Input: part model. Units: mm. Frame: model coordinates. A direction names the side the tool comes from. Coordinates: 2 decimals unless noted, no trailing zeros. Write each loop counter-clockwise with the first axis right and the second up, starting at its lowest first coordinate (ties: lowest second). Pieces come first, ordered by that corner, then holes. Notation, with made-up numbers: M -17.5,39 L 38.5,39 A10 ccw 38.5,56 Z; hole C -23.5,42 d7. An arc over 180 degrees is marked long. Use CSV: the item, a comma, the result in double quotes.
```python
from build123d import *

# Parameters (mm, degrees)
SKETCH_1_W                  = 40
SKETCH_1_H                  = 47.1
EXTRUDE_1_DEPTH             = 10
HOLE_WIZARD_M4_1_AT_2_COUNT = 2
HOLE_WIZARD_M4_1_AT_2_PITCH = 32
HOLE_WIZARD_M5_1_D          = 4.2
HOLE_WIZARD_M5_1_DEPTH      = 12.4
HOLE_WIZARD_M5_1_TIP        = 1.2618073
CUT_EXTRUDE_1_REACH         = 34.475
SKETCH_8_W                  = 24
SKETCH_8_H                  = 27.1
FILLET_1_R                  = 3


with BuildPart() as part:
    # 草图1 → 凸台-拉伸1 (new body)
    with BuildSketch(Plane.XY):
        Rectangle(SKETCH_1_W, SKETCH_1_H)
    extrude(amount=EXTRUDE_1_DEPTH)

    # 草图4 → M4 螺纹孔1 (revolve, cut)
    with BuildSketch(Plane(origin=(-16, 23.55, 5), x_dir=(0, 0, 1), z_dir=(1, 0, 0))):
        Polygon((0, 0), (0, 11.091420021), (1.65, 10.1), (1.65, 0), align=None)
    hole_wizard_m4_1 = revolve(axis=Axis((-16, 29.9, 5), (0, -1, 0)), mode=Mode.SUBTRACT)

    # M4 螺纹孔1 at 2: M4 螺纹孔1 ×2
    with Locations(*[(i * HOLE_WIZARD_M4_1_AT_2_PITCH, 0, 0) for i in range(1, HOLE_WIZARD_M4_1_AT_2_COUNT)]):
        add(hole_wizard_m4_1, mode=Mode.SUBTRACT)

    # 镜向1: M4 螺纹孔1 across plane
    add(hole_wizard_m4_1.mirror(Plane.ZX), mode=Mode.SUBTRACT)

    # 镜向1 copy 1 sketch → 镜向1 copy 1 (revolve, cut)
    with BuildSketch(Plane(origin=(16, -23.55, 5), x_dir=(0, 0, 1), z_dir=(1, 0, 0))):
        Polygon((0, 0), (0, -11.091420021), (1.65, -10.1), (1.65, 0), align=None)
    revolve(axis=Axis((16, -29.9, 5), (0, -1, 0)), mode=Mode.SUBTRACT)

    # M5 螺纹孔1
    with Locations(Plane.XY.offset(10)):
        with Locations((0, 0)):
            Hole(HOLE_WIZARD_M5_1_D / 2, depth=HOLE_WIZARD_M5_1_DEPTH)
            with Locations((0, 0, -(HOLE_WIZARD_M5_1_DEPTH + HOLE_WIZARD_M5_1_TIP / 2))):  # 118° drill point
                Cone(0, HOLE_WIZARD_M5_1_D / 2, HOLE_WIZARD_M5_1_TIP, mode=Mode.SUBTRACT)

    # 切除-拉伸1: up to this face of the body (flat: up to its plane)
    cut_extrude_1_end = Plane(part.part.faces().sort_by_distance((0, -22.932067156, 0))[0])
    # 草图8 → 切除-拉伸1 (cut, up to the picked face)
    with BuildSketch(Plane.XY.offset(10), mode=Mode.PRIVATE) as cut_extrude_1_sk1:
        with Locations((20, 0)):
            Rectangle(SKETCH_8_W, SKETCH_8_H)
    cut_extrude_1_tool1 = split(extrude(cut_extrude_1_sk1.sketch, amount=-CUT_EXTRUDE_1_REACH, mode=Mode.PRIVATE), bisect_by=cut_extrude_1_end, keep=Keep.BOTH, mode=Mode.PRIVATE)
    cut_extrude_1 = cut_extrude_1_tool1.solids().sort_by(Axis((20, 0, 10), (0, 0, -1)))[0]
    add(cut_extrude_1, mode=Mode.SUBTRACT)

    # 镜向2: 切除-拉伸1 across plane
    add(cut_extrude_1.mirror(Plane(origin=(0, 0, 0), x_dir=(0, 0, 1), z_dir=(1, 0, 0))), mode=Mode.SUBTRACT)

    # 圆角1
    fillet_1_edges = [part.edges().sort_by_distance(p)[0] for p in [
        (8, 13.55, 5),
        (8, -13.55, 5),
        (-8, -13.55, 5),
        (-8, 13.55, 5),
    ]]
    fillet(fillet_1_edges, radius=FILLET_1_R)


solid = part.part
```
1. Section C-C (z = 7.5). Return loops of the section in (x, y).
Resolved:
outline,"M -20,-23.55 L 20,-23.55 L 20,-13.55 L 11,-13.55 A3 cw 8,-10.55 L 8,10.55 A3 cw 11,13.55 L 20,13.55 L 20,23.55 L -20,23.55 L -20,13.55 L -11,13.55 A3 cw -8,10.55 L -8,-10.55 A3 cw -11,-13.55 L -20,-13.55 Z; hole C 0,0 d4.2"
2. Section A-A (x = 0). Return loops of the section in (y, z), then the cut area to 3 significant figures.
Resolved:
outline,"M -23.55,0 L -2.1,0 L -2.1,10 L -23.55,10 Z; M 2.1,0 L 23.55,0 L 23.55,10 L 2.1,10 Z"
area,"429 mm^2"
3. Section D-D (x = 16). Return loops of the section in (y, z), then the cut area to 3 significant figures.
Resolved:
outline,"M -23.55,0 L -13.55,0 L -13.55,3.35 L -23.55,3.35 Z; M -23.55,6.65 L -13.55,6.65 L -13.55,10 L -23.55,10 Z; M 13.55,0 L 23.55,0 L 23.55,3.35 L 13.55,3.35 Z; M 13.55,6.65 L 23.55,6.65 L 23.55,10 L 13.55,10 Z"
area,"134 mm^2"
4. Material intervals for line 1 (X direction, y = 17, z = 5); line 2 (Y direction, x = -12, z = 1); line 3 (Z direction, x = 16, y = -15.5), sorted ascending. Write a range as [from, to].
Resolved:
line 1,"x = [-20, -17.65], [-14.35, 14.35], [17.65, 20]"
line 2,"y = [-23.55, -13.55], [13.55, 23.55]"
line 3,"z = [0, 3.35], [6.65, 10]"
5. Access query for faces 5 (the flat face through (-20, -19, 5)), 6 (the flat face through (14, 13.55, 6)), 7 (the cylindrical face through (-8.9, -12.69, 4.93)). Directions: +Z, -Z, +X, -X, +Y, -Y. A direction counts if a zero-diameter tool reaches every point of the face in a straight line with its end or side. Return the directions, or none.
Resolved:
face 5,"+Z, -Z, -X, +Y, -Y"
face 6,"+Z, -Z, +X"
face 7,"+Z, -Z, -X"
6. Contact query for flat-ended pins moving along their axis: pin 1 Ø1 at (y, z) = (7.5, 2) entering from -X; pin 2 Ø3 at (y, z) = (-2.5, 3) entering from +X. Output: stop coordinate, or through.
Resolved:
pin 1,"stops at x = -8"
pin 2,"stops at x = 8"
7. Mould query, pull axis Z, two halves, no side actions, for faces 1 (the cylindrical face through (-16.07, -18.62, 3.35)), 2 (the flat face through (4, 0, 10)), 3 (the flat face through (-14, -13.55, 6)), 4 (the cylindrical face through (-16.07, 18.62, 3.35)). Classes: pulls with the +Z half, pulls with the -Z half, needs draft (parallel to the pull), parting line crosses it, or undercut.
Resolved:
face 1,"undercut"
face 2,"pulls with the +Z half"
face 3,"needs draft"
face 4,"undercut"
8. Section B-B (y = 0). Return loops of the section in (x, z), then the cut area to 3 significant figures.
Resolved:
outline,"M -8,0 L -2.1,0 L -2.1,10 L -8,10 Z; M 2.1,0 L 8,0 L 8,10 L 2.1,10 Z"
area,"118 mm^2"
